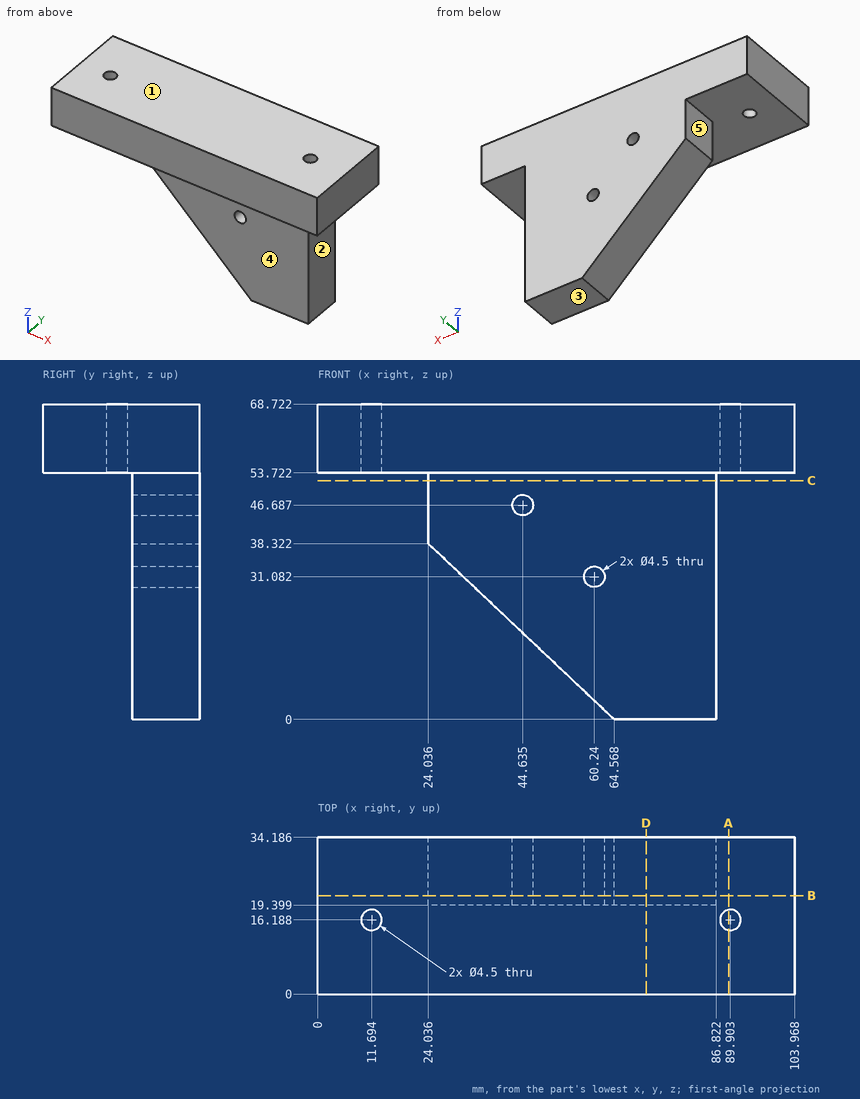
Job drawing, mm, ordinate dimensions from the low corner. One solid piece. A direction names the side the tool comes from. Round coordinates to 2 decimals unless told otherwise and drop trailing zeros. Loops run counter-clockwise (first coordinate to the right, second up) from the corner with the lowest first, then second, coordinate; pieces in that order, holes last.
Item 1: Cut at D-D, the plane x = 71.5. Give the cut face in (y, z).
Item 2: Drill centre lines: line 1 (Y direction, x = 53, z = 36); line 2 (Z direction, x = 6, y = 28); line 3 (X direction, y = 29.5, z = 40) (1 decimal). Where is each one in solid material? Low to high.
Item 3: 3-axis set-ups, long thin cutter, end or side, ignore diameter. For the marked faces 1, 2, 3, 4 and 5: which of +Z, -Z, +X, -X, +Y, -Y reach the whole face in a straight line?
Item 4: Cut at B-B, the plane y = 21.5. State how many separate pieces and enclosed holes the cut face has, then the cut area to 3 significant figures.
Item 5: Drop flat-ended pins along their axis: P1, Ø6, axis at x = 11.69, y = 16.19, coming from the -Z side; P2, Ø8, axis at y = 21, z = 45.5, coming from the +X side; P3, Ø1.5, axis at x = 35.5, z = 43.5, coming from the -Y side. Give the stop position or say it passes through.
Item 6: Cut at A-A, the plane x = 89.5. Give the cut face in (y, z) (1 decimal).
Item 7: Cut at C-C, the plane z = 52. Give the cut face in (x, y) (1 decimal).
A:
1. outline: (0, 53.72) - (19.4, 53.72) - (19.4, 0) - (34.19, 0) - (34.19, 68.72) - (0, 68.72) - close
2. line 1: y = 19.4 to 34.19
2. line 2: z = 53.72 to 68.72
2. line 3: x = 24 to 86.8
3. face 1: +Z, +X, -X, +Y, -Y
3. face 2: -Z, +X, +Y, -Y
3. face 3: -Z, +X, -X, +Y, -Y
3. face 4: -Z, +X, -X, -Y
3. face 5: -Z, -X, +Y, -Y
4. separate pieces: 1
4. enclosed holes: 2
4. area: 4,120 mm2
5. P1: stops at z = 53.72
5. P2: stops at x = 86.82
5. P3: stops at y = 19.4
6. outline: (0, 53.7) - (14, 53.7) - (14, 68.7) - (0, 68.7) - close; (18.4, 53.7) - (34.2, 53.7) - (34.2, 68.7) - (18.4, 68.7) - close
7. outline: (24, 19.4) - (86.8, 19.4) - (86.8, 34.2) - (24, 34.2) - close
